For this review, take the finished solid that the model builds, in its own axes (mm). A direction names the side the tool comes from. Coordinates: 2 decimals unless noted, no trailing zeros. Order: outer loops, then holes, each group sorted by start corner. A loop starts at its lowest first (then second) coordinate and runs counter-clockwise, first axis right, second up.
from build123d import *

# Parameters (mm, degrees)
F0_W     = 10
F0_H     = 10
F1_DEPTH = 41
F2_W     = 10
F2_H     = 35
F3_DEPTH = 7
F4_R     = 1.35
F5_DEPTH = 50


with BuildPart() as f1:
    # F0 (on Top) → F1 (new body)
    with BuildSketch(Plane.XY):
        Rectangle(F0_W, F0_H)
    extrude(amount=F1_DEPTH)

    # F2 (on face) → F3 (cut)
    with BuildSketch(Plane.XZ.offset(5)):
        with Locations((0, 20.5)):
            Rectangle(F2_W, F2_H)
    extrude(amount=-F3_DEPTH, mode=Mode.SUBTRACT)

    # F4 (on face) → F5 (cut)
    with BuildSketch(Plane.XY.offset(41)):
        with Locations((0, -1.5)):
            Circle(F4_R)
    extrude(amount=-F5_DEPTH, mode=Mode.SUBTRACT)


solid = f1.part
1. Clearance check with flat-ended pins moving along their axes: pin 1 Ø3 at (x, z) = (2.5, 24) entering from -Y; pin 2 Ø3.5 at (x, y) = (0, -1.5) entering from -Z. State where each tip first meets the part, or that it passes through.
Answer below:
pin 1: stops at y = 2
pin 2: stops at z = 0
2. Take a section at C-C, the plane x = -3.75. Give the boundary of the cut face in (y, z).
Answer below:
outline: (-5, 0) - (5, 0) - (5, 41) - (-5, 41) - (-5, 38) - (2, 38) - (2, 3) - (-5, 3) - close
3. Take a section at D-D, the plane z = 13.5. Give the boundary of the cut face in (x, y).
Answer below:
outline: (-5, 2) - (5, 2) - (5, 5) - (-5, 5) - close
4. Take a section at B-B, the plane y = -1.5. Give the boundary of the cut face in (x, z).
Answer below:
outline: (-5, 0) - (-1.35, 0) - (-1.35, 3) - (-5, 3) - close; (-5, 38) - (-1.35, 38) - (-1.35, 41) - (-5, 41) - close; (1.35, 0) - (5, 0) - (5, 3) - (1.35, 3) - close; (1.35, 38) - (5, 38) - (5, 41) - (1.35, 41) - close
5. The part is to be moulded in two halves that separate along X. For faces 1 (the face through (-5, 2.2, 20.2)), 2 (the face through (-0.176, -0.161, 39.521)), 3 (the face through (-0.1, 0, 38)), 4 (the face through (-0.176, -0.161, 1.521)), say which applies: +X half, -X half, draft (parallel to the pull), parting line (faces both ways), or undercut.
Answer below:
face 1: -X half
face 2: undercut
face 3: draft
face 4: undercut
6. Take a section at A-A, the plane x = 0. Give the boundary of the cut face in (y, z).
Answer below:
outline: (-5, 0) - (-2.85, 0) - (-2.85, 3) - (-5, 3) - close; (-5, 38) - (-2.85, 38) - (-2.85, 41) - (-5, 41) - close; (-0.15, 0) - (5, 0) - (5, 41) - (-0.15, 41) - (-0.15, 38) - (2, 38) - (2, 3) - (-0.15, 3) - close
7. To check wall thickness, follow L1, parallel to Z at x = -2.25, y = -1; L2, parallel to Y at x = 0, z = 39.8; L3, parallel to Y at x = -1.75, z = 37. State the ranges of each line that lie inside material, in increasing order.
Answer below:
L1: z = 0 to 3, 38 to 41
L2: y = -5 to -2.85, -0.15 to 5
L3: y = 2 to 5
8. Machinability: for faces 5 (the face through (0, 5, 20)), 6 (the face through (0, 2, 21)), which of the approach directions +Z, -Z, +X, -X, +Y, -Y give a long, thin tool a straight path to every point of the face, cutting with its end or side? Answer none if there is none.
Answer below:
face 5: +Z, -Z, +X, -X, +Y
face 6: +X, -X, -Y
